```python
from build123d import *
from build123d.topology import SkipClean

# Parameters (mm, degrees)
SKETCH1_R                       = 5
SKETCH1_R_2                     = 3
BOSS_EXTRUDE1_DEPTH             = 3
SKETCH2_R                       = 5
SKETCH2_R_2                     = 4
BOSS_EXTRUDE2_DEPTH             = 16
BOSS_EXTRUDE3_DEPTH             = 10
CUT_EXTRUDE1_DEPTH              = 16
SKETCH5_R                       = 4
CUT_EXTRUDE2_DEPTH              = 18
CUT_EXTRUDE3_DEPTH              = 30
SKETCH8_W                       = 6
SKETCH8_H                       = 6
CUT_EXTRUDE4_DEPTH              = 7
SKETCH9_R                       = 3
CUT_EXTRUDE5_DEPTH              = 7
BOSS_EXTRUDE4_START             = 20
SKETCH10_R                      = 4
SKETCH10_R_2                    = 3
BOSS_EXTRUDE4_DEPTH             = 20
BOSS_EXTRUDE5_REACH             = 25.135
BOSS_EXTRUDE5_END_RADIUS        = 4
SKETCH11_R                      = 2
BOSS_EXTRUDE5_DIRECTION_2_DEPTH = 1.5
FILLET1_R                       = 0.4


with BuildPart() as part:
    # Sketch1 → Boss-Extrude1 (new body)
    with BuildSketch(Plane(origin=(0, 0, 0), x_dir=(1, 0, 0), z_dir=(0, 1, 0))):
        with Locations(Location((0, 0, 0), (0, 0, 270))):
            Circle(SKETCH1_R)
        with Locations(Location((0, 0, 0), (0, 0, 270))):
            Circle(SKETCH1_R_2, mode=Mode.SUBTRACT)
    extrude(amount=BOSS_EXTRUDE1_DEPTH)

    # Sketch2 → Boss-Extrude2 (add)
    with BuildSketch(Plane(origin=(0, 3, 0), x_dir=(1, 0, 0), z_dir=(0, 1, 0))):
        with Locations(Location((0, 0, 0), (0, 0, 270))):
            Circle(SKETCH2_R)
        with Locations(Location((0, 0, 0), (0, 0, 270))):
            Circle(SKETCH2_R_2, mode=Mode.SUBTRACT)
    extrude(amount=BOSS_EXTRUDE2_DEPTH)

    # Sketch3 → Boss-Extrude3 (add)
    with BuildSketch(Plane(origin=(5, 0, 0), x_dir=(0, 0, -1), z_dir=(1, 0, 0))):
        with BuildLine():
            Line((7, 4), (0, 4))
            Line((0, 4), (0, 8.807417596))
            ThreePointArc((0, 8.807417596), (11.245917567, 17.68240924), (7, 4))
        make_face()
    extrude(amount=-BOSS_EXTRUDE3_DEPTH)

    # Sketch4 → Cut-Extrude1 (cut)
    with BuildSketch(Plane(origin=(5, 0, 0), x_dir=(0, 0, -1), z_dir=(1, 0, 0))):
        with BuildLine():
            Line((-5, 11.5), (-9.7286492, 16.2286492))
            Line((-9.7286492, 16.2286492), (-5.44277466, 22.641996471))
            Line((-5.44277466, 22.641996471), (7, 19))
            add(Edge.make_bspline(
                [(7, 19), (6.318131306, 19.000028418), (1.657993515, 18.351162216), (-3.360726674, 13.19986781), (-5, 11.5)],
                knots=[0, 0, 0, 0, 0.141151098, 1, 1, 1, 1], degree=3))
        make_face()
    extrude(amount=-CUT_EXTRUDE1_DEPTH, mode=Mode.SUBTRACT)

    # Sketch5 → Cut-Extrude2 (cut)
    with BuildSketch(Plane(origin=(0, 3, 0), x_dir=(1, 0, 0), z_dir=(0, 1, 0))):
        with Locations(Location((0, 0, 0), (0, 0, 90))):
            Circle(SKETCH5_R)
    extrude(amount=CUT_EXTRUDE2_DEPTH, mode=Mode.SUBTRACT)

    # Sketch7 → Cut-Extrude3 (cut)
    with BuildSketch(Plane(origin=(0, 3, 0), x_dir=(1, 0, 0), z_dir=(0, 1, 0))):
        Polygon((0, 0), (-3.75, 0), (-3.75, 16.160631513), (3.75, 16.160631513), (3.75, 0), align=None)
    extrude(amount=CUT_EXTRUDE3_DEPTH, mode=Mode.SUBTRACT)

    # Sketch8 → Cut-Extrude4 (cut)
    with BuildSketch(Plane(origin=(5, 0, 0), x_dir=(0, 0, -1), z_dir=(1, 0, 0))):
        with Locations((7, 11.5)):
            Rectangle(SKETCH8_W, SKETCH8_H)
    extrude(amount=-CUT_EXTRUDE4_DEPTH, mode=Mode.SUBTRACT)

    # Sketch9 → Cut-Extrude5 (cut)
    with BuildSketch(Plane.ZY.offset(5)):
        with Locations((-7, 11.5)):
            Circle(SKETCH9_R)
    extrude(amount=-CUT_EXTRUDE5_DEPTH, mode=Mode.SUBTRACT)

    # Sketch10 → Boss-Extrude4 (add)
    with SkipClean():  # the faces are left unmerged after this step: merging them gives an invalid solid
        with BuildSketch(Plane.XZ.offset(BOSS_EXTRUDE4_START)):
            with Locations(Location((0, 0, 0), (0, 0, 90))):
                Circle(SKETCH10_R)
            with Locations(Location((0, 0, 0), (0, 0, 270))):
                Circle(SKETCH10_R_2, mode=Mode.SUBTRACT)
        extrude(amount=-BOSS_EXTRUDE4_DEPTH)

    # Boss-Extrude5: up to this cylinder (the profile starts outside it)
    with SkipClean():  # the faces are left unmerged after this step: merging them gives an invalid solid
        boss_extrude5_end = Plane(origin=(0, -16, 0), z_dir=(0, 1, 0)) * Cylinder(BOSS_EXTRUDE5_END_RADIUS, 59.27, mode=Mode.PRIVATE)
        # Sketch11 → Boss-Extrude5 (add, up to the surface)
        with BuildSketch(Plane.XY.offset(-4), mode=Mode.PRIVATE) as boss_extrude5_sk1:
            with Locations((0, -16)):
                Circle(SKETCH11_R)
        boss_extrude5_tool1 = extrude(boss_extrude5_sk1.sketch, amount=BOSS_EXTRUDE5_REACH, mode=Mode.PRIVATE) - boss_extrude5_end
        add(boss_extrude5_tool1.solids().sort_by_distance((0, -16, -4))[0])
        add(boss_extrude5_tool1.solids().sort_by_distance((0, -16, -4))[1])

    # Sketch11 → Boss-Extrude5 direction 2 (add)
    with SkipClean():  # the faces are left unmerged after this step: merging them gives an invalid solid
        with BuildSketch(Plane.XY.offset(-4)):
            with Locations((0, -16)):
                Circle(SKETCH11_R)
        extrude(amount=-BOSS_EXTRUDE5_DIRECTION_2_DEPTH)

    # Fillet1
    fillet1_edges = [part.edges().sort_by_distance(p)[0] for p in [
        (-2, -16, -5.5),
    ]]
    fillet(fillet1_edges, radius=FILLET1_R)


solid = part.part
```
The listing builds one solid part. Answer for the finished solid, in the listing's coordinates (mm). A direction names the side the tool comes from. Give positions to 0.01 mm unless a question says otherwise; leave off trailing zeros. Order: outer loops, then holes, each group sorted by start corner. A loop starts at its lowest first (then second) coordinate and runs counter-clockwise, first axis right, second up. Notation, with made-up numbers: M 18,68.5 L 68,68.5 A20 cw 68,95.5 Z; hole C -2,6.5 d5. An arc over 180 degrees is marked long. Put each result on its own line as item: value. Start each with the question number.
Item 1: The part is cut by section C-C, the plane y = -8.5. Determine the outline of the cut face in (x, z).
Item 2: For a pull along X with two mould halves and no side action, classify faces 4 (the face through (-4.38, 10.35, -4.23)), 5 (the face through (5, 11.6, -3.8)), 6 (the face through (-3.75, 9, -9)) as +X half, -X half, draft (parallel to the pull), parting line (faces both ways), or undercut.
Item 3: The part is cut by section A-A, the plane y = 5.5. Determine the outline of the cut face in (x, z), and give its area (3 significant figures).
Item 4: The part is cut by section B-B, the plane z = -12. Determine the outline of the cut face in (x, y).
Item 5: Find the intervals of material crossed by line 1 along X through (y, z) = (11.75, 0); line 2 along X through (y, z) = (6.5, -8.5); line 3 along Y through (x, z) = (-4.7, -7), in increasing order.
Item 6: Which of the six approach directions +Z, -Z, +X, -X, +Y, -Y give full straight-line access (tool end or side, diameter ignored) to faces 1 (the face through (4, 4, -4)), 2 (the face through (4, 11, -10)), 3 (the face through (3.75, 11, -11))?
Item 7: Flat-ended cylindrical pins translate along their axes: P1, Ø5, axis at x = 2, z = -2, coming from the -Y side; P2, Ø2, axis at y = -13, z = 2, coming from the -X side; P3, Ø0.6, axis at x = 4.5, y = 11.5, coming from the +Z side; P4, Ø1.6, axis at x = 0, y = -16, coming from the -Z side. Find the tip coordinate at first contact, or state that the pin passes through.
Answer key:
1. outline: C 0,0 d8; hole C 0,0 d6
2. face 4: draft
2. face 5: +X half
2. face 6: undercut
3. outline: M -5,-11.5 L -3.75,-11.5 L -3.75,-1.39 A4 cw long 3.75,-1.39 L 3.75,-11.5 L 5,-11.5 L 5,0 A5 ccw -5,0 Z
3. area: 42.4 mm²
4. outline: M -5,5.91 L -3.75,5.91 L -3.75,17.09 L -5,17.09 Z; M 3.75,5.91 L 5,5.91 L 5,17.09 L 3.75,17.09 Z
5. line 1: x = -5 to -4, 4 to 5
5. line 2: x = -5 to -3.75, 3.75 to 5
5. line 3: y = 4 to 8.5, 14.5 to 19
6. face 1: -Z, +X, -Y
6. face 2: +X
6. face 3: -Z, +Y
7. P1: stops at y = -20
7. P2: stops at x = -3.87
7. P3: stops at z = 2.71
7. P4: stops at z = -5.5
